```python
from build123d import *

# Parameters (mm, degrees)
BASE_EXTRUDE_DEPTH = 3


with BuildPart() as part:
    # Sketch1 → Base-Extrude (new body)
    with BuildSketch(Plane.XY):
        with BuildLine():
            Line((905.965375708, -110.41468189), (908.594990659, -110.41468189))
            ThreePointArc((908.594990659, -110.41468189), (909.468405337, -100.295175968), (907.11402855, -90.41468189))
            Line((907.11402855, -90.41468189), (876.335760757, -90.41468189))
            ThreePointArc((876.335760757, -90.41468189), (874.726506158, -100.41468189), (876.335760757, -110.41468189))
            Line((876.335760757, -110.41468189), (878.965375708, -110.41468189))
            Line((878.965375708, -110.41468189), (878.965375708, -101.027413417))
            Line((878.965375708, -101.027413417), (881.965375708, -101.027413417))
            Line((881.965375708, -101.027413417), (881.965375708, -110.41468189))
            Line((881.965375708, -110.41468189), (892.465375708, -110.41468189))
            Line((892.465375708, -110.41468189), (902.965375708, -110.41468189))
            Line((902.965375708, -110.41468189), (902.965375708, -101.027413417))
            Line((902.965375708, -101.027413417), (905.965375708, -101.027413417))
            Line((905.965375708, -101.027413417), (905.965375708, -110.41468189))
        make_face()
    extrude(amount=BASE_EXTRUDE_DEPTH)


solid = part.part
```
Build history of the part. All positions in model axes, mm. A direction names the side the tool comes from. Round coordinates to 2 decimals unless told otherwise and drop trailing zeros. Loops run counter-clockwise (first coordinate to the right, second up) from the corner with the lowest first, then second, coordinate; pieces in that order, holes last. Notation, with made-up numbers: M 79.25,76.25 L 124.25,76.25 A15 cw 124.25,90.25 Z; hole C 83.25,75.25 d8. An arc over 180 degrees is marked long. Answer as CSV lines item,"result".
1. Cut at C-C on x = 879.5. Write the cut outline in (y, z).
Resolved:
outline,"M -101.03,0 L -90.41,0 L -90.41,3 L -101.03,3 Z"
2. Wall check: probe 1 along X at (y, z) = (-105.25, 2.05); probe 2 along X at (y, z) = (-103.75, 1); probe 3 along Y at (x, z) = (881.5, 0.25). Give the ranges that are in metal, low to high. Write a range as [from, to].
Resolved:
probe 1,"x = [875.1, 878.97], [881.97, 902.97], [905.97, 909.45]"
probe 2,"x = [874.9, 878.97], [881.97, 902.97], [905.97, 909.54]"
probe 3,"y = [-101.03, -90.41]"
3. Cut at A-A on y = -108.75. Write the cut outline in (x, z), then the cut area to 3 significant figures.
Resolved:
outline,"M 875.84,0 L 878.97,0 L 878.97,3 L 875.84,3 Z; M 881.97,0 L 902.97,0 L 902.97,3 L 881.97,3 Z; M 905.97,0 L 908.97,0 L 908.97,3 L 905.97,3 Z"
area,"81.4 mm²"
4. 3-axis set-ups, long thin cutter, end or side, ignore diameter. For faces 1 (the flat face through (881.965, -106, 1)), 2 (the flat face through (907, -110.415, 1)): which of +Z, -Z, +X, -X, +Y, -Y reach the whole face in a straight line?
Resolved:
face 1,"+Z, -Z, -Y"
face 2,"+Z, -Z, +X, -X, -Y"
5. Cut at B-B on z = 1.25. Write the cut outline in (x, y) (3 decimals), then the cut area to 3 significant figures.
Resolved:
outline,"M 876.336,-110.415 L 878.965,-110.415 L 878.965,-101.027 L 881.965,-101.027 L 881.965,-110.415 L 902.965,-110.415 L 902.965,-101.027 L 905.965,-101.027 L 905.965,-110.415 L 908.595,-110.415 A31.875 ccw 907.114,-90.415 L 876.336,-90.415 A31.875 ccw Z"
area,"617 mm²"
6. Flat gauge pins, fed straight in: P1, Ø0.9, axis at x = 905, z = 2, coming from the -Y side; P2, Ø1.5, axis at y = -93, z = 0.5, coming from the +X side; P3, Ø1.5, axis at y = -107.5, z = 2, coming from the -X side. Where does each tip first touch, or does it go through?
Resolved:
P1,"stops at y = -101.03"
P2,"stops at x = 908.29"
P3,"stops at x = 875.36"
7. Two-plate mould, pull along X, no slides. Class faces 3 (the cylindrical face through (874.727, -100.272, 1.479)), 4 (the flat face through (878, -110.415, 1)), 5 (the flat face through (880, -101.027, 1)): released by +X, released by -X, zero draft, split by the parting line, or undercut.
Resolved:
face 3,"released by -X"
face 4,"zero draft"
face 5,"undercut"
8. Cut at D-D on y = -102.5. Write the cut outline in (x, z).
Resolved:
outline,"M 874.79,0 L 878.97,0 L 878.97,3 L 874.79,3 Z; M 881.97,0 L 902.97,0 L 902.97,3 L 881.97,3 Z; M 905.97,0 L 909.56,0 L 909.56,3 L 905.97,3 Z"
